Read the model definition and answer for the solid it produces. Units are mm, in the model's axes. A direction names the side the tool comes from. Coordinates: 2 decimals unless noted, no trailing zeros. Write each loop counter-clockwise with the first axis right and the second up, starting at its lowest first coordinate (ties: lowest second). Pieces come first, ordered by that corner, then holes.
(1) The part is cut by section A-A, the plane z = 7. Determine the outline of the cut face in (x, y).
(2) Determine the mould class of faces 1 (the flat face through (-38.1, 1, 2)), 2 (the flat face through (38.1, 1, 2)), 3 (the cylindrical face through (28.028, 10.864, 2.493)), 4 (the flat face through (-1, -13.615, 1)) for opening direction X: pulls with the +X half, pulls with the -X half, needs draft (parallel to the pull), parting line crosses it, or undercut.
(3) The part is cut by section B-B, the plane x = 3.5. Determine the outline of the cut face in (y, z), and give its area (3 significant figures).
(4) The part is cut by section C-C, the plane y = 9.5. Determine the outline of the cut face in (x, z), and give its area (3 significant figures).
(5) Straight lines are drawn through the part: line 1 along Y through (x, z) = (-28.57, 2.75); line 2 along X through (y, z) = (0, 6.75); line 3 along Z through (x, y) = (21.5, -1). For each, find the intervals that lie inside material, in ascending order.
(6) Which of the six approach directions +Z, -Z, +X, -X, +Y, -Y give full straight-line access (tool end or side, diameter ignored) to faces 5 (the flat face through (-29, 12, 2)), 6 (the flat face through (-1, -7, 3)), 7 (the flat face through (-1, 10, 3))?
(7) Given pin 1 (8 mm diameter, centred on x = -28.57, y = -10.06, fed in from -Z); pin 2 (1 mm diameter, centred on x = -30, y = -6, fed in from +Z); pin 3 (1.2 mm diameter, centred on x = -28.57, y = 13.3, fed in from +Z); pin 4 (4 mm diameter, centred on x = 28.57, y = -10.06, fed in from +Z), each flat-ended and moving along its own axis, determine where each tip first touches the part or whether it passes through.
```python
from build123d import *

# Parameters (mm, degrees)
F0_W          = 76.2
F0_H          = 30.48
F0_R          = 2.5
F2_DEPTH      = 3
F0_R_2        = 1
F3_DEPTH      = 2
F4_START      = 28.1
F4_DEPTH      = 10
F5_START      = -28.1
F5_DEPTH      = 10
F6_DEPTH      = 28.1
F6_DEPTH_BACK = 28.1
F7_R          = 1


with BuildPart() as f2:
    # F0 (on Top) → F2 (new body)
    with BuildSketch(Plane.XY):
        with Locations((0, 1.624652555)):
            Rectangle(F0_W, F0_H)
        with Locations((-28.57, -10.055347445)):
            Circle(F0_R, mode=Mode.SUBTRACT)
        with Locations((28.57, -10.055347445)):
            Circle(F0_R, mode=Mode.SUBTRACT)
        with Locations((-28.57, 13.304652555)):
            Circle(F0_R, mode=Mode.SUBTRACT)
        with Locations((28.57, 13.304652555)):
            Circle(F0_R, mode=Mode.SUBTRACT)
    extrude(amount=F2_DEPTH)

    # F0 (on Top) → F3 (join)
    with BuildSketch(Plane.XY):
        with Locations((28.57, 13.304652555)):
            Circle(F0_R)
        with Locations((28.57, 13.304652555)):
            Circle(F0_R_2, mode=Mode.SUBTRACT)
        with Locations((28.57, -10.055347445)):
            Circle(F0_R)
        with Locations((28.57, -10.055347445)):
            Circle(F0_R_2, mode=Mode.SUBTRACT)
        with Locations((-28.57, -10.055347445)):
            Circle(F0_R)
        with Locations((-28.57, -10.055347445)):
            Circle(F0_R_2, mode=Mode.SUBTRACT)
        with Locations((-28.57, 13.304652555)):
            Circle(F0_R)
        with Locations((-28.57, 13.304652555)):
            Circle(F0_R_2, mode=Mode.SUBTRACT)
    extrude(amount=F3_DEPTH)

    # F1 (on Right) → F4 (join)
    with BuildSketch(Plane.YZ.offset(F4_START)):
        with BuildLine():
            ThreePointArc((-1.3122499903, 5.5619300567), (-2.4969921778, 3.8736281168), (-4.365347445, 3))
            Line((-4.365347445, 3), (-0.6014154225, 3))
            ThreePointArc((-0.6014154225, 3), (-1.2561375211, 4.1979197446), (-1.3122499903, 5.5619300567))
        make_face()
        with BuildLine():
            Line((3.8707205325, 3), (7.634652555, 3))
            ThreePointArc((7.634652555, 3), (5.7662972877, 3.8736281168), (4.5815551003, 5.5619300567))
            ThreePointArc((4.5815551003, 5.5619300567), (4.6213486925, 5.2822165518), (4.634652555, 5))
            ThreePointArc((4.634652555, 5), (4.4371696319, 3.9295337307), (3.8707205325, 3))
        make_face()
        with BuildLine():
            ThreePointArc((-1.3122499903, 5.5619300567), (-1.2561375211, 4.1979197446), (-0.6014154225, 3))
            Line((-0.6014154225, 3), (3.8707205325, 3))
            ThreePointArc((3.8707205325, 3), (4.4371696319, 3.9295337307), (4.634652555, 5))
            ThreePointArc((4.634652555, 5), (4.6213486925, 5.2822165518), (4.5815551003, 5.5619300567))
            ThreePointArc((4.5815551003, 5.5619300567), (1.634652555, 8), (-1.3122499903, 5.5619300567))
        make_face()
        with BuildLine():
            ThreePointArc((1.634652555, 4), (0.9275457738, 5.7071067812), (2.634652555, 5))
            ThreePointArc((2.634652555, 5), (2.3417593362, 4.2928932188), (1.634652555, 4))
        make_face(mode=Mode.SUBTRACT)
    extrude(amount=F4_DEPTH)

    # F1 (on Right) → F5 (join)
    with BuildSketch(Plane.YZ.offset(F5_START)):
        with BuildLine():
            ThreePointArc((-1.3122499903, 5.5619300567), (-2.4969921778, 3.8736281168), (-4.365347445, 3))
            Line((-4.365347445, 3), (-0.6014154225, 3))
            ThreePointArc((-0.6014154225, 3), (-1.2561375211, 4.1979197446), (-1.3122499903, 5.5619300567))
        make_face()
        with BuildLine():
            Line((3.8707205325, 3), (7.634652555, 3))
            ThreePointArc((7.634652555, 3), (5.7662972877, 3.8736281168), (4.5815551003, 5.5619300567))
            ThreePointArc((4.5815551003, 5.5619300567), (4.6213486925, 5.2822165518), (4.634652555, 5))
            ThreePointArc((4.634652555, 5), (4.4371696319, 3.9295337307), (3.8707205325, 3))
        make_face()
        with BuildLine():
            ThreePointArc((-1.3122499903, 5.5619300567), (-1.2561375211, 4.1979197446), (-0.6014154225, 3))
            Line((-0.6014154225, 3), (3.8707205325, 3))
            ThreePointArc((3.8707205325, 3), (4.4371696319, 3.9295337307), (4.634652555, 5))
            ThreePointArc((4.634652555, 5), (4.6213486925, 5.2822165518), (4.5815551003, 5.5619300567))
            ThreePointArc((4.5815551003, 5.5619300567), (1.634652555, 8), (-1.3122499903, 5.5619300567))
        make_face()
        with BuildLine():
            ThreePointArc((1.634652555, 4), (0.9275457738, 5.7071067812), (2.634652555, 5))
            ThreePointArc((2.634652555, 5), (2.3417593362, 4.2928932188), (1.634652555, 4))
        make_face(mode=Mode.SUBTRACT)
    extrude(amount=-F5_DEPTH)

    # F1 (on Right) → F6 (cut, two sides)
    with BuildSketch(Plane.YZ) as f6_sk:
        with BuildLine():
            Line((3.8707205325, 3), (-0.6014154225, 3))
            ThreePointArc((-0.6014154225, 3), (1.634652555, 2), (3.8707205325, 3))
        make_face()
    extrude(amount=-F6_DEPTH, mode=Mode.SUBTRACT)
    extrude(f6_sk.sketch, amount=F6_DEPTH_BACK, mode=Mode.SUBTRACT)

    # F7
    f7_edges = [f2.edges().sort_by_distance(p)[0] for p in [
        (38.1, -13.615347, 1.5),
        (38.1, 16.864653, 1.5),
        (-38.1, 16.864653, 1.5),
        (-38.1, -13.615347, 1.5),
    ]]
    fillet(f7_edges, radius=F7_R)


solid = f2.part
```
Computed:
1. outline: (-38.1, -0.6) - (-28.1, -0.6) - (-28.1, 3.87) - (-38.1, 3.87) - close; (28.1, -0.6) - (38.1, -0.6) - (38.1, 3.87) - (28.1, 3.87) - close
2. face 1: pulls with the -X half
2. face 2: pulls with the +X half
2. face 3: undercut
2. face 4: needs draft
3. outline: (-13.62, 0) - (16.86, 0) - (16.86, 3) - (3.87, 3) arc R3 cw to (-0.6, 3) - (-13.62, 3) - close
3. area: 88.3 mm2
4. outline: (-38.1, 0) - (38.1, 0) - (38.1, 3) - (-38.1, 3) - close
4. area: 229 mm2
5. line 1: y = -13.62 to -12.56, -7.56 to 10.8, 15.8 to 16.86
5. line 2: x = -38.1 to -28.1, 28.1 to 38.1
5. line 3: z = 0 to 3
6. face 5: +Z
6. face 6: +Z, -Y
6. face 7: +Z, +Y
7. pin 1: stops at z = 0
7. pin 2: stops at z = 3
7. pin 3: passes through
7. pin 4: stops at z = 2
